Check sheet for the modelled part. Datum: model origin and axes. Units: mm. A direction names the side the tool comes from. Give positions to 0.01 mm unless a question says otherwise; leave off trailing zeros. Use a Markdown table: item, result. Add a question column.
1. Set-up check for faces 1 (the flat face through (36, 3, -6)), 2 (the flat face through (-23.794, 0, -6)), 3 (the flat face through (26.206, 0, -6)): record each of +Z, -Z, +X, -X, +Y, -Y from which the full face is reachable in a straight line by a thin tool's end or side.
2. Release check for a two-part mould opening along X. For faces 4 (the flat face through (-14, 0, -12)), 5 (the flat face through (9, 0, 0)), 6 (the flat face through (45.206, 0, -6)), 7 (the flat face through (-4.794, 0, -6)) record: released by +X, released by -X, zero draft, split by the parting line, or undercut.
3. Gauge pin test, flat ends, axial feed: P1, Ø3, axis at y = 0, z = -5.5, coming from the +X side; P2, Ø6, axis at x = 22.5, y = 0, coming from the -Z side; P3, Ø3.5, axis at x = 40, z = -6, coming from the -Y side. Record the tip position at first contact, or that the pin passes through.
4. Scan lines: probe 1 along X at (y, z) = (-1.5, -4.5); probe 2 along Y at (x, z) = (2, 29); probe 3 along Y at (x, z) = (58, 50.5). Record each from-to range of solid material in increasing order. Write a range as [from, to].
from build123d import *

# Parameters (mm, degrees)
F5_W     = 19
F5_H     = 12
F6_DEPTH = 3


with BuildPart() as f3:
    # F0 (on Front) → F3 section 0
    with BuildSketch(Plane.XZ):
        with BuildLine():
            add(Edge.make_bspline(
                [(-33.4539487958, 0), (-33.4539475141, 0), (1.8967446088, 54.4877709826), (87.6792873597, 91.6592373474), (104.7614702217, 65.474297534), (62.0720738186, 52.2220753998), (65.4690045649, 12.016653457), (66.9079050422, 0)],
                knots=[0, 0, 0, 0, 0.2258859795, 0.5122183994, 0.6229913169, 0.7959413028, 1, 1, 1, 1], degree=3))
            Line((-33.4539487958, 0), (66.9079050422, 0))
        make_face()
    # F2 (on offset) → F3 section 1
    with BuildSketch(Plane.XZ.offset(5)):
        with BuildLine():
            add(Edge.make_bspline(
                [(-12.3913707212, 0), (-4.3907383925, 10.8659039807), (5.5855721966, 32.4205796435), (83.1861544033, 82.0508925585), (76.9843234234, 65.810450768), (58.1651473267, 60.4997302931), (1.3900142987, 9.9120248782), (0, 0)],
                knots=[0, 0, 0, 0, 0.2108575974, 0.4883367114, 0.5577546823, 0.7117913524, 1, 1, 1, 1], degree=3))
            Line((-12.3913707212, 0), (0, 0))
        make_face()
    loft()

    # F4: F3 across plane


with BuildPart() as f3_1:
    add(f3.part)
    add(f3.part.mirror(Plane.XZ))

    # F5 (on Front) → F6 (join, symmetric)
    with BuildSketch(Plane.XZ):
        with Locations((35.7055166066, -6)):
            Rectangle(F5_W, F5_H)
        with Locations((-14.2944833934, -6)):
            Rectangle(F5_W, F5_H)
    extrude(amount=F6_DEPTH, both=True)


solid = f3_1.part
Worked answers:
| question | item | result |
|---|---|---|
| 1 | face 1 | -Z, +X, -X, +Y |
| 1 | face 2 | -Z, -X, +Y, -Y |
| 1 | face 3 | -Z, +Y, -Y |
| 2 | face 4 | zero draft |
| 2 | face 5 | undercut |
| 2 | face 6 | released by +X |
| 2 | face 7 | undercut |
| 3 | P1 | stops at x = 45.21 |
| 3 | P2 | stops at z = 0 |
| 3 | P3 | stops at y = -3 |
| 4 | probe 1 | x = [-23.79, -4.79], [26.21, 45.21] |
| 4 | probe 2 | y = [-3.02, 3.02] |
| 4 | probe 3 | y = [-3.4, 3.4] |
